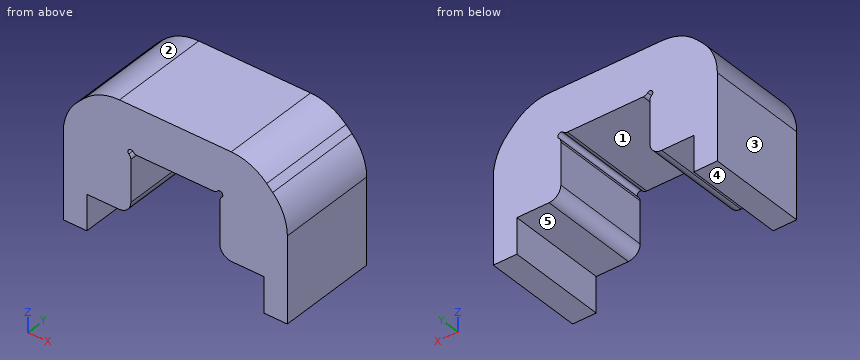
Autodesk Fusion 360 part; units mm, degrees
sketch "Sketch1" plane through (0, 0, 0) normal (0, 1, 0) x (1, 0, 0)
  line L0 (0, 0) -> (4, 0)
  line L1 (4, 0) -> (4, -6)
  line L2 (4, -6) -> (11.45, -6)
  line L3 (11.45, -6) -> (11.45, -16.2)
  line L4 (11.45, -16.2) -> (26.55, -16.2)
  line L5 (26.55, -16.2) -> (26.55, -6)
  line L6 (26.55, -6) -> (34, -6)
  line L7 (34, -6) -> (34, 0)
  line L8 (34, 0) -> (38, 0)
  line L9 (38, 0) -> (38, -24)
  line L10 (38, -24) -> (0, -24)
  line L11 (0, -24) -> (0, 0)
  dimension "d1" = 15.1
  dimension "d2" = 10.2
  dimension "d3" = 30
  dimension "d4" = 6
  dimension "d5" = 4
  dimension "d6" = 24
extrude "Extrude1" add sketch "Sketch1" along normal blind 17
chamfer "Chamfer1" distance 6 distance2 6 2 edges at (38, 8.5, 24) (0, 8.5, 24) measured on face at (25.3333, 5.6667, 24) measured on face at (0, 5.6667, 16)
fillet "Fillet1" radius 2 2 edges at (11.45, 8.5, 6) (26.55, 8.5, 6)
sketch "Sketch2" plane through (0, 0, 0) normal (0, -1, 0) x (1, 0, 0)
  arc A0 (26.55, 8) -> (28.55, 6) centre (28.55, 8) ccw
  line L0 (28.55, 6) -> (34, 6)
  line L1 (34, 6) -> (34, 0)
  line L2 (34, 0) -> (38, 0)
  line L3 (38, 0) -> (38, 18)
  line L4 (38, 18) -> (32, 24)
  line L5 (32, 24) -> (6, 24)
  line L6 (6, 24) -> (0, 18)
  line L7 (0, 18) -> (0, 0)
  line L8 (0, 0) -> (4, 0)
  line L9 (4, 0) -> (4, 6)
  line L10 (4, 6) -> (9.45, 6)
  arc A1 (9.45, 6) -> (11.45, 8) centre (9.45, 8) ccw
  line L11 (11.45, 8) -> (11.45, 16.2)
  line L12 (11.45, 16.2) -> (26.55, 16.2)
  line L13 (26.55, 16.2) -> (26.55, 8)
  circle A2 centre (11.45, 16.2) radius 0.5
  circle A3 centre (26.55, 16.2) radius 0.5
  dimension "d13" = 1
  dimension "d14" = 1
extrude "Extrude2" cut sketch "Sketch2" against normal through all contours L12 L13 A3 | L11 L12 A2 picked at (26.2406, 16.3214) picked at (11.3772, 15.8756)
fillet "Fillet2" radius 1 4 edges at (11.45, 8.5, 15.7) (11.95, 8.5, 16.2) (26.05, 8.5, 16.2) (26.55, 8.5, 15.7)
fillet "Fillet5" radius 8.5 4 edges at (6, 8.5, 24) (0, 8.5, 18) (32, 8.5, 24) (38, 8.5, 18)
For this review, take the finished solid that the model builds, in its own axes (mm). Face numbers are marked on the shaded views. A direction names the side the tool comes from. Round coordinates to 2 decimals unless told otherwise and drop trailing zeros. Loops run counter-clockwise (first coordinate to the right, second up) from the corner with the lowest first, then second, coordinate; pieces in that order, holes last. Notation, with made-up numbers: (53, 27.5) - (74, 27.5) arc R20 ccw to (74, 48.5) - close; hole circle Ø9 at (67, 66.5). An arc over 180 degrees is marked (long way). One line per item, written item: value. Start each with the question number.
Item 1: Take a section at C-C (x = 15). Give the boundary of the cut face in (y, z), plus the area to 3 significant figures.
Item 2: The part is to be moulded in two halves that separate along X. For the marked faces 3, 4 and 5, say which applies: +X half, -X half, draft (parallel to the pull), parting line (faces both ways), or undercut.
Item 3: Take a section at D-D (z = 21). Give the boundary of the cut face in (x, y).
Item 4: For L1, parallel to X at y = 13.75, z = 13.5; L2, parallel to X at y = 11, z = 3.5; L3, parallel to Z at x = 14.5, y = 13.75, list the stretches that pass through material, from the lowest coordinate up.
Item 5: For the marked faces 1 and 2, list the 3-axis set-ups (+Z, -Z, +X, -X, +Y, -Y) from which the entire face can be reached by the end or side of a thin tool; tool diameter is ignored.
Item 6: Clearance check with flat-ended pins moving along their axes: pin 1 Ø4.5 at (x, y) = (7, 11.5) entering from -Z; pin 2 Ø1.8 at (y, z) = (12, 2) entering from -X; pin 3 Ø2 at (y, z) = (13, 16.5) entering from +X; pin 4 Ø4 at (x, y) = (20, 9) entering from -Z. State where each tip first meets the part, or that it passes through.
Item 7: Take a section at B-B (y = 3). Give the boundary of the cut face in (x, z).
Item 8: Take a section at A-A (z = 13.5). Give the boundary of the cut face in (x, y), plus the area to 3 significant figures.
Answer below:
1. outline: (0, 16.2) - (17, 16.2) - (17, 24) - (0, 24) - close
1. area: 133 mm2
2. face 3: -X half
2. face 4: draft
2. face 5: undercut
3. outline: (3, 0) - (35, 0) - (35, 17) - (3, 17) - close
4. L1: x = 0 to 11.45, 26.55 to 38
4. L2: x = 0 to 4, 34 to 38
4. L3: z = 16.2 to 24
5. face 1: -Z, +Y, -Y
5. face 2: +Z, -X, +Y, -Y
6. pin 1: stops at z = 6
6. pin 2: stops at x = 0
6. pin 3: stops at x = 37.94
6. pin 4: stops at z = 16.2
7. outline: (0, 0) - (4, 0) - (4, 6) - (9.45, 6) arc R2 ccw to (11.45, 8) - (11.45, 15.08) arc R1 ccw to (11.12, 15.83) arc R0.5 cw (long way) to (11.82, 16.53) arc R1 ccw to (12.57, 16.2) - (25.43, 16.2) arc R1 ccw to (26.18, 16.53) arc R0.5 cw (long way) to (26.88, 15.83) arc R1 ccw to (26.55, 15.08) - (26.55, 8) arc R2 ccw to (28.55, 6) - (34, 6) - (34, 0) - (38, 0) - (38, 14.48) arc R8.5 ccw to (35.51, 20.49) - (34.49, 21.51) arc R8.5 ccw to (28.48, 24) - (9.52, 24) arc R8.5 ccw to (3.51, 21.51) - (2.49, 20.49) arc R8.5 ccw to (0, 14.48) - close
8. outline: (0, 0) - (11.45, 0) - (11.45, 17) - (0, 17) - close; (26.55, 0) - (38, 0) - (38, 17) - (26.55, 17) - close
8. area: 389 mm2
